Design review of the part built by this model. Coordinates are the model's own, in mm. A direction names the side the tool comes from. Coordinates: 2 decimals unless noted, no trailing zeros. Write each loop counter-clockwise with the first axis right and the second up, starting at its lowest first coordinate (ties: lowest second). Pieces come first, ordered by that corner, then holes. Notation, with made-up numbers: (64, 73) - (111, 73) arc R31 cw to (111, 104) - close; hole circle Ø8 at (13, -36). An arc over 180 degrees is marked (long way). Answer as a JSON object with one key per item and string values.
```python
from build123d import *

# Parameters (mm, degrees)
F0_W      = 20
F0_H      = 20
F1_DEPTH  = 10
F2_T      = -3
F3_R      = 7
F4_DEPTH  = 6
F5_W      = 14
F5_H      = 14
F6_DEPTH  = 6
F8_DEPTH  = 6
F10_DEPTH = 6


with BuildPart() as f1:
    # F0 (on Front) → F1 (new body, symmetric)
    with BuildSketch(Plane.XZ):
        Rectangle(F0_W, F0_H)
    extrude(amount=F1_DEPTH, both=True)

    # F2
    f2_openings = [f1.faces().sort_by_distance(p)[0] for p in [
        (0, 0, 10),
    ]]
    offset(amount=F2_T, openings=f2_openings)

    # F3 (on face) → F4 (cut)
    with BuildSketch(Plane(origin=(0, 10, 0), x_dir=(-1, 0, 0), z_dir=(0, 1, 0))):
        Circle(F3_R)
    extrude(amount=-F4_DEPTH, mode=Mode.SUBTRACT)

    # F5 (on face) → F6 (cut)
    with BuildSketch(Plane.XZ.offset(10)):
        Rectangle(F5_W, F5_H)
    extrude(amount=-F6_DEPTH, mode=Mode.SUBTRACT)

    # F7 (on face) → F8 (cut)
    with BuildSketch(Plane.YZ.offset(10)):
        Polygon((-0.240179, 0), (-7, -7), (7, -7), (0.240179, 0), (7, 7), (-7, 7), align=None)
    extrude(amount=-F8_DEPTH, mode=Mode.SUBTRACT)

    # F9 (on face) → F10 (cut)
    with BuildSketch(Plane(origin=(-10, 0, 0), x_dir=(0, -1, 0), z_dir=(-1, 0, 0))):
        with BuildLine():
            ThreePointArc((7, 7), (-2.899495, 2.899495), (-7, -7))
            Line((-7, -7), (7, -7))
            Line((7, -7), (7, 7))
        make_face()
    extrude(amount=-F10_DEPTH, mode=Mode.SUBTRACT)


solid = f1.part
```
(1) The part is to be moulded in two halves that separate along Y. For faces 1 (the face through (9, 0, 7)), 2 (the face through (-2, 10, 7)), 3 (the face through (0, 0, -10)), say which applies: pulls with the +Y half, pulls with the -Y half, needs draft (parallel to the pull), parting line crosses it, or undercut.
Solved:
{"face 1": "undercut", "face 2": "pulls with the +Y half", "face 3": "needs draft"}
(2) Take a section at D-D, the plane x = 7.5. Write out the cut boundary in (y, z), and give its area (3 significant figures).
Solved:
{"outline": "(-10, -10) - (10, -10) - (10, 10) - (-10, 10) - close; hole (-7, -7) - (7, -7) - (0.24, 0) - (7, 7) - (-7, 7) - (-0.24, 0) - close", "area": "299 mm^2"}
(3) For pin 1 (2 mm diameter, centred on x = 4.5, z = -4.5, fed in from -Y); pin 2 (2 mm diameter, centred on y = 2.5, z = 0.5, fed in from -X), all flat-tipped, find the tip position at first contact; note any pin that passes through.
Solved:
{"pin 1": "stops at y = 7", "pin 2": "stops at x = 7"}
(4) To check wall thickness, follow line 1 (X direction, y = 8.55, z = 0). State the ranges of the line that lie inside material, in increasing order. Write a range as from..to.
Solved:
{"line 1": "x = -10..-7, 7..10"}
(5) Tool access review of faces 4 (the face through (-8.5, 2.8, 3)), 5 (the face through (-7, -9, 0)), 6 (the face through (8.52, -3.57, -3.45)): name each direction out of +Z, -Z, +X, -X, +Y, -Y from which nothing blocks a thin tool from reaching the whole face with its end or side.
Solved:
{"face 4": "-X", "face 5": "-Y", "face 6": "+X, -X"}
(6) Take a section at B-B, the plane y = 5. Write out the cut boundary in (x, z).
Solved:
{"outline": "(-10, -10) - (10, -10) - (10, -7) - (-10, -7) - close; (-10, 0.21) - (-7, 0.21) - (-7, 10) - (-10, 10) - close; (7, -4.93) - (10, -4.93) - (10, 4.93) - (7, 4.93) - close; (7, 7) - (10, 7) - (10, 10) - (7, 10) - close"}
(7) Take a section at A-A, the plane x = -2. Write out the cut boundary in (y, z).
Solved:
{"outline": "(-10, -10) - (10, -10) - (10, -6.71) - (7, -6.71) - (7, -7) - (-10, -7) - close; (-10, 7) - (-7, 7) - (-7, 10) - (-10, 10) - close; (7, 6.71) - (10, 6.71) - (10, 10) - (7, 10) - close"}
(8) Take a section at C-C, the plane z = -4.25. Write out the cut boundary in (x, y), and give its area (3 significant figures).
Solved:
{"outline": "(-10, -10) - (-7, -10) - (-7, -7) - (-10, -7) - close; (-10, 6.73) - (-7, 6.73) - (-7, 7) - (-5.56, 7) - (-5.56, 10) - (-10, 10) - close; (5.56, 7) - (7, 7) - (7, 4.34) - (10, 4.34) - (10, 10) - (5.56, 10) - close; (7, -10) - (10, -10) - (10, -4.34) - (7, -4.34) - close", "area": "61.4 mm^2"}
